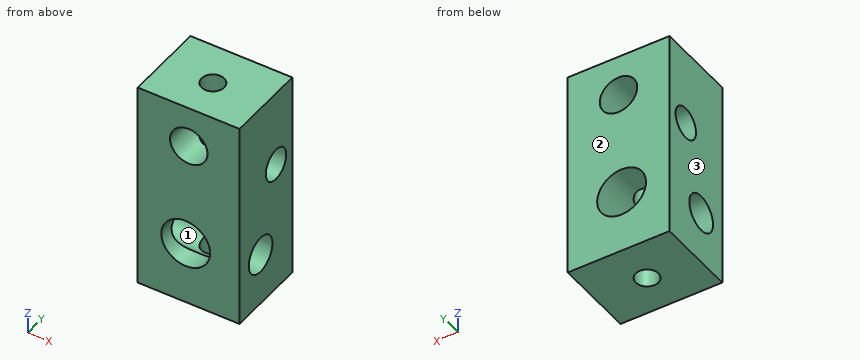
from build123d import *

# Parameters (mm, degrees)
F0_W     = 48.24812
F0_H     = 100.085393
F1_DEPTH = 38.735
F2_R     = 8.875977
F3_DEPTH = 72.39
F4_R     = 11.577097
F5_DEPTH = 81.915
F6_R     = 7.510162
F6_R_2   = 8.700388
F7_DEPTH = 74.295
F8_R     = 5.377664
F9_DEPTH = 137.795


with BuildPart() as f1:
    # F0 (on Front) → F1 (new body)
    with BuildSketch(Plane.XZ):
        with Locations((24.12406, 50.042696)):
            Rectangle(F0_W, F0_H)
    extrude(amount=F1_DEPTH)

    # F2 (on face) → F3 (cut)
    with BuildSketch(Plane.XZ.offset(38.735)):
        with Locations((24.177499, 80.580726)):
            Circle(F2_R)
    extrude(amount=-F3_DEPTH, mode=Mode.SUBTRACT)

    # F4 (on face) → F5 (cut)
    with BuildSketch(Plane.XZ.offset(38.735)):
        with Locations((22.72643, 30.099884)):
            Circle(F4_R)
    extrude(amount=-F5_DEPTH, mode=Mode.SUBTRACT)

    # F6 (on face) → F7 (cut)
    with BuildSketch(Plane.YZ.offset(48.24812)):
        with Locations((-11.938325, 63.61071)):
            Circle(F6_R)
        with Locations((-23.248304, 25.008034)):
            Circle(F6_R_2)
    extrude(amount=-F7_DEPTH, mode=Mode.SUBTRACT)

    # F8 (on face) → F9 (cut)
    with BuildSketch(Plane.XY.offset(100.085393)):
        with Locations((23.553871, -20.061549)):
            Circle(F8_R)
    extrude(amount=-F9_DEPTH, mode=Mode.SUBTRACT)


solid = f1.part
Can you work these out from the model? Positions are in its coordinate system, mm. Face numbers are marked on the shaded views. Coordinates: 2 decimals unless noted, no trailing zeros. Order: outer loops, then holes, each group sorted by start corner. A loop starts at its lowest first (then second) coordinate and runs counter-clockwise, first axis right, second up. Notation, with made-up numbers: M -3,83 L 10,83 A17 cw 10,109 Z; hole C 10.5,38 d7. An arc over 180 degrees is marked long. Write item = value, one per line.
(1) Suppose I cut it at C-C on z = 22.5. Please give me the cut outline in (x, y) (3 decimals).
Results are:
outline = M 0,-38.735 L 13.993,-38.735 L 13.993,-31.579 L 0,-31.579 Z; M 0,-14.917 L 13.993,-14.917 L 13.993,0 L 0,0 Z; M 31.46,-38.735 L 48.248,-38.735 L 48.248,-31.579 L 31.46,-31.579 Z; M 31.46,-14.917 L 48.248,-14.917 L 48.248,0 L 31.46,0 Z
(2) If we mould it in two halves opening along Y, with no side actions, what happens to the marked faces 1, 2 and 3? For each: pulls with the +Y half, pulls with the -Y half, needs draft (parallel to the pull), parting line crosses it, or undercut.
Results are:
face_1 = undercut
face_2 = pulls with the +Y half
face_3 = needs draft
(3) Suppose I cut it at B-B on x = 16.5. Please give me the cut outline in (y, z) (3 decimals).
Results are:
outline = M -38.735,0 L 0,0 L 0,20.34 L -15.906,20.34 A8.7 cw -30.59,20.34 L -38.735,20.34 Z; M -38.735,39.86 L 0,39.86 L 0,76.127 L -38.735,76.127 Z; M -38.735,85.035 L 0,85.035 L 0,100.085 L -38.735,100.085 Z; hole C -11.938,63.611 d15.02
(4) I need wall thicknesses on line 1 along Z through (x, y) = (16, -29.5); line 2 along Z through (x, y) = (26.5, -1.5); line 3 along Y through (x, z) = (4.5, 28) (3 decimals). Which ranges of each line are inside material? Lowest first, please. Write a range as [from, to].
Results are:
line_1 = [0, 18.96], [39.52, 77.13], [84.03, 100.09]
line_2 = [0, 19.16], [41.04, 72.01], [89.15, 100.09]
line_3 = [-38.735, -31.418], [-15.079, 0]
(5) Suppose I cut it at A-A on y = -29. Please give me the cut outline in (x, z).
Results are:
outline = M 0,0 L 48.25,0 L 48.25,18.48 L 0,18.48 Z; M 0,31.54 L 11.24,31.54 A11.58 cw 34.21,31.54 L 48.25,31.54 L 48.25,100.09 L 0,100.09 Z; hole C 24.18,80.58 d17.75
(6) Suppose I cut it at D-D on y = -7.5. Please give me the cut outline in (x, z).
Results are:
outline = M 0,0 L 48.25,0 L 48.25,57.55 L 0,57.55 Z; M 0,69.67 L 48.25,69.67 L 48.25,100.09 L 0,100.09 Z; hole C 22.73,30.1 d23.15; hole C 24.18,80.58 d17.75
